Geometry check sheet. Reference: the model listing, model coordinates, mm. A direction names the side the tool comes from. Give positions to 0.01 mm unless a question says otherwise; leave off trailing zeros. Order: outer loops, then holes, each group sorted by start corner. A loop starts at its lowest first (then second) coordinate and runs counter-clockwise, first axis right, second up. Notation, with made-up numbers: M -10,46 L 40,46 A21 ccw 40,77 Z; hole C 22,-2.75 d1. An arc over 180 degrees is marked long. Answer as CSV lines item,"result". Start each with the question number.
Q1. Set-up check for faces 4 (the flat face through (115, 3, -15.031)), 5 (the flat face through (-78.397, 3, -24)), 6 (the flat face through (-63, 3, 54.838)): record each of +Z, -Z, +X, -X, +Y, -Y from which the full face is reachable in a straight line by a thin tool's end or side.
Q2. Mould release check, pull along Z, two halves, no side actions. Record for faces 1 (the flat face through (17, 3, 61.188)), 2 (the flat face through (-46.647, 3, 58)), 3 (the flat face through (-78.397, 3, 1)): +Z half, -Z half, draft (parallel to the pull), parting line (faces both ways), or undercut.
Q3. Section check A-A, the plane x = -70.5. Record the boundary of the cut face in (y, z).
Q4. Go/stop test with flat-tipped pins: pin 1 (3 mm diameter, centred on x = -82, y = 4, fed in from +Z); pin 2 (3 mm diameter, centred on x = 116, y = 2.5, fed in from +Z); pin 3 (3 mm diameter, centred on y = 2, z = 1, fed in from -X). Record where each tip stops, or that it passes through.
Q5. Thickness scan on line 1 (X direction, y = 0.5, z = 55); line 2 (X direction, y = 2.5, z = 12.5); line 3 (Z direction, x = -5, y = 3.25). Record the ranges inside material, lowest first.
Q6. Section check B-B, the plane z = -38.5. Record the boundary of the cut face in (x, y), then the cut area to 3 significant figures.
```python
from build123d import *

# Parameters (mm, degrees)
SKETCH1_W           = 203.2
SKETCH1_H           = 107.95
BOSS_EXTRUDE1_DEPTH = 6.35
SKETCH2_W           = 38.1
SKETCH2_H           = 6.35
SKETCH2_W_2         = 25.4
CUT_EXTRUDE1_DEPTH  = 7.35
SKETCH3_W           = 6.35
SKETCH3_H           = 6.35
CUT_EXTRUDE2_DEPTH  = 7.35


with BuildPart() as part:
    # Sketch1 → Boss-Extrude1 (new body)
    with BuildSketch(Plane(origin=(0, 0, 0), x_dir=(1, 0, 0), z_dir=(0, 1, 0))):
        with Locations((16.852621149, -7.21321811)):
            Rectangle(SKETCH1_W, SKETCH1_H)
    extrude(amount=BOSS_EXTRUDE1_DEPTH)

    # Sketch2 → Cut-Extrude1 (cut, through all)
    with BuildSketch(Plane(origin=(0, 6.35, 0), x_dir=(1, 0, 0), z_dir=(0, 1, 0))):
        with Locations((99.402621149, -58.01321811)):
            Rectangle(SKETCH2_W, SKETCH2_H)
        with Locations((42.252621149, -58.01321811)):
            Rectangle(SKETCH2_W_2, SKETCH2_H)
        with Locations((-8.547378851, -58.01321811)):
            Rectangle(SKETCH2_W_2, SKETCH2_H)
        with Locations((-65.697378851, -58.01321811)):
            Rectangle(SKETCH2_W, SKETCH2_H)
    extrude(amount=-CUT_EXTRUDE1_DEPTH, mode=Mode.SUBTRACT)

    # Sketch3 → Cut-Extrude2 (cut, through all)
    with BuildSketch(Plane(origin=(0, 6.35, 0), x_dir=(1, 0, 0), z_dir=(0, 1, 0))):
        with Locations((115.277621149, -45.31321811)):
            Rectangle(SKETCH3_W, SKETCH3_H)
        with Locations((115.277621149, -32.61321811)):
            Rectangle(SKETCH3_W, SKETCH3_H)
        with Locations((115.277621149, -19.91321811)):
            Rectangle(SKETCH3_W, SKETCH3_H)
        with Locations((115.277621149, -7.194250827)):
            Rectangle(SKETCH3_W, SKETCH3_H)
        with Locations((115.277621149, 5.505749173)):
            Rectangle(SKETCH3_W, SKETCH3_H)
        with Locations((115.277621149, 18.205749173)):
            Rectangle(SKETCH3_W, SKETCH3_H)
        with Locations((115.277621149, 30.905749173)):
            Rectangle(SKETCH3_W, SKETCH3_H)
        with Locations((115.277621149, 43.605749173)):
            Rectangle(SKETCH3_W, SKETCH3_H)
        with Locations((-81.572378851, -51.66321811)):
            Rectangle(SKETCH3_W, SKETCH3_H)
        with Locations((-81.572378851, -38.96321811)):
            Rectangle(SKETCH3_W, SKETCH3_H)
        with Locations((-81.572378851, -26.26321811)):
            Rectangle(SKETCH3_W, SKETCH3_H)
        with Locations((-81.572378851, -13.56321811)):
            Rectangle(SKETCH3_W, SKETCH3_H)
        with Locations((-81.572378851, -0.86321811)):
            Rectangle(SKETCH3_W, SKETCH3_H)
        with Locations((-81.572378851, 11.83678189)):
            Rectangle(SKETCH3_W, SKETCH3_H)
        with Locations((-81.572378851, 24.53678189)):
            Rectangle(SKETCH3_W, SKETCH3_H)
        with Locations((-81.572378851, 37.23678189)):
            Rectangle(SKETCH3_W, SKETCH3_H)
    extrude(amount=-CUT_EXTRUDE2_DEPTH, mode=Mode.SUBTRACT)


solid = part.part
```
Answer block:
1,face 4,"+X, +Y, -Y"
1,face 5,"-X, +Y, -Y"
1,face 6,"+Z, -X, +Y, -Y"
2,face 1,"+Z half"
2,face 2,"draft"
2,face 3,"undercut"
3,outline,"M 0,-46.76 L 6.35,-46.76 L 6.35,54.84 L 0,54.84 Z"
4,pin 1,"stops at z = 48.49"
4,pin 2,"stops at z = 54.84"
4,pin 3,"stops at x = -78.4"
5,line 1,"x = -46.65 to -21.25, 4.15 to 29.55, 54.95 to 80.35"
5,line 2,"x = -78.4 to 118.45"
5,line 3,"z = -46.76 to 54.84"
6,outline,"M -78.4,0 L 118.45,0 L 118.45,6.35 L -78.4,6.35 Z"
6,area,"1,250 mm2"
